Could you check a few things on this drawing? It's one solid part, dimensions in mm from its lowest x, y, z. A direction names the side the tool comes from. Round coordinates to 2 decimals unless told otherwise and drop trailing zeros. Loops run counter-clockwise (first coordinate to the right, second up) from the corner with the lowest first, then second, coordinate; pieces in that order, holes last. Notation, with made-up numbers: (6.25, 46) -> (29.25, 46) arc R11 ccw to (29.25, 55) -> close; hole circle Ø11 at (-24.5, 74.25). An arc over 180 degrees is marked (long way). Put each result on its own line as item: value. Start each with the question number.
1. Imagine slicing it at A-A, the plane y = 22.25. Please give me the cut outline in (x, z) (3 decimals).
2. Imagine slicing it at C-C, the plane x = 52. Please give me the cut outline in (y, z) (3 decimals), and give its area (3 significant figures).
3. Which directions (+Z, -Z, +X, -X, +Y, -Y) give clear straight access to the entire face, cutting with the end or side of a thin tool? Please do the marked faces 1 and 2.
4. I need wall thicknesses on line 1 (Z direction, x = 152, y = 4.5); line 2 (X direction, y = 21.5, z = 153) (3 decimals). Which ranges of each line are inside material? Lowest first, please. Write a range as [from, to].
5. Imagine slicing it at D-D, the plane y = 6.75. Count the separate pieces of the cut face and the enclosed holes in it, and give its area (3 significant figures).
6. Imagine slicing it at B-B, the plane z = 251. Please give me the cut outline in (x, y) (3 decimals).
7. I'm going to push flat-ended pins straight in: P1, Ø6.5, axis at x = 168.275, z = 269.875, coming from the -Y side; P2, Ø12, axis at x = 41.5, z = 34, coming from the +Y side (3 decimals); P3, Ø4, axis at x = 162.5, z = 237.5, coming from the +Y side (3 decimals); P4, Ø2, axis at x = 156, y = 16, coming from the +Z side. Where does each tip first touch, or does it pass through?
8. If we mould it in two halves opening along X, with no side actions, what happens to the marked faces 3 and 4? For each: pulls with the +X half, pulls with the -X half, needs draft (parallel to the pull), parting line crosses it, or undercut.
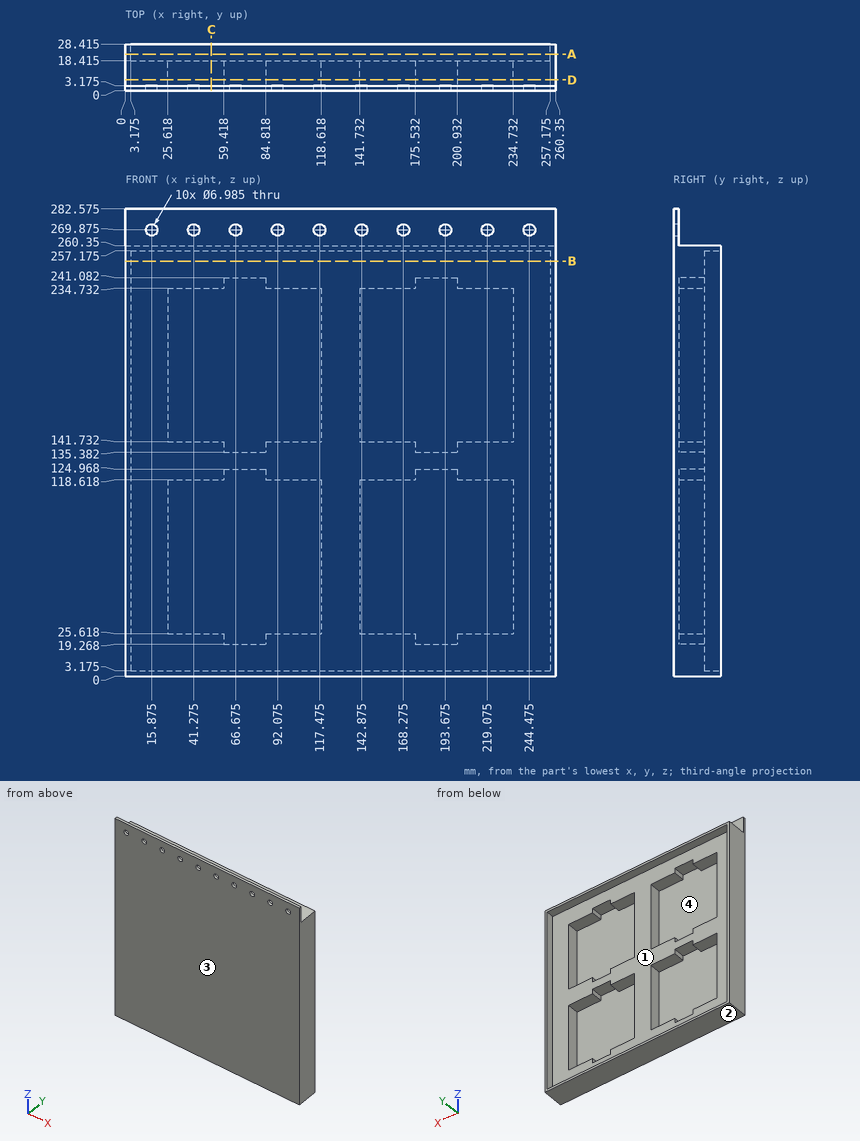
Entries:
1. outline: (0, 0) -> (260.35, 0) -> (260.35, 260.35) -> (0, 260.35) -> close; hole (3.175, 3.175) -> (257.175, 3.175) -> (257.175, 257.175) -> (3.175, 257.175) -> close
2. outline: (0, 0) -> (28.415, 0) -> (28.415, 3.175) -> (18.415, 3.175) -> (18.415, 25.618) -> (3.175, 25.618) -> (3.175, 118.618) -> (18.415, 118.618) -> (18.415, 141.732) -> (3.175, 141.732) -> (3.175, 234.732) -> (18.415, 234.732) -> (18.415, 257.175) -> (28.415, 257.175) -> (28.415, 260.35) -> (3.175, 260.35) -> (3.175, 282.575) -> (0, 282.575) -> close
2. area: 2,090 mm^2
3. face 1: +Y
3. face 2: -Z, +X, -X, +Y, -Y
4. line 1: [0, 25.62], [118.62, 141.73], [234.73, 260.35]
4. line 2: [0, 3.175], [257.175, 260.35]
5. separate pieces: 1
5. enclosed holes: 4
5. area: 31,900 mm^2
6. outline: (0, 0) -> (260.35, 0) -> (260.35, 28.415) -> (257.175, 28.415) -> (257.175, 18.415) -> (3.175, 18.415) -> (3.175, 28.415) -> (0, 28.415) -> close
7. P1: through
7. P2: y = 3.175
7. P3: y = 18.415
7. P4: z = 260.35
8. face 3: needs draft
8. face 4: undercut
